from build123d import *

# Parameters (mm, degrees)
F1_W     = 50.8
F1_H     = 50.8
F3_W     = 50.8
F3_H     = 50.8
F4_DEPTH = 660.4


with BuildPart() as f2:
    # F2: sweep along a path in F0
    with BuildLine(Plane.XY) as f2_path:
        Line((0, 0), (0, 762))
        Line((0, 762), (1219.2, 762))
        Line((1219.2, 762), (1219.2, 0))
        Line((1219.2, 0), (0, 0))
    # F1 (on Front) → F2 (sweep)
    with BuildSketch(Plane.XZ):
        with Locations((25.4, -25.4)):
            Rectangle(F1_W, F1_H)
    sweep(path=f2_path.line, transition=Transition.RIGHT)

    # F3 (on face) → F4 (join, through all)
    with BuildSketch(Plane.XZ.offset(-711.2)):
        with Locations((990.6, -25.4)):
            Rectangle(F3_W, F3_H)
    extrude(amount=F4_DEPTH)


solid = f2.part
Source: CAD feature listing. Evaluate the final solid. Frame: model axes, mm. A direction names the side the tool comes from. Give positions to 0.01 mm unless a question says otherwise; leave off trailing zeros. Write each loop counter-clockwise with the first axis right and the second up, starting at its lowest first coordinate (ties: lowest second). Pieces come first, ordered by that corner, then holes. Notation, with made-up numbers: M 54.5,8.5 L 112.5,8.5 A16 cw 112.5,39.5 Z; hole C 68,-23.75 d1. An arc over 180 degrees is marked long. Return JSON: item names as keys, results as strings. Group by question number.
1) Set-up query: faces 5 (the face through (1093, 711.2, -26)), 6 (the face through (968, 383, -50.8)). Return all of +Z, -Z, +X, -X, +Y, -Y with unobstructed straight access to the full face (end or side cutting, diameter ignored); none if empty.
2) Cut plane B-B, the plane y = 316. Output: boundary loops of the cut face in (x, z).
3) Draft query along Y for faces 1 (the face through (974, 355, 0)), 2 (the face through (618, 762, -25)), 3 (the face through (601, 0, -25)), 4 (the face through (1016, 386, -26)). Return one class per face: released by +Y, released by -Y, zero draft, split by the parting line, or undercut.
4) Cut plane C-C, the plane z = -38. Output: boundary loops of the cut face in (x, y), then the cut area to 3 significant figures.
5) Ray query, L1, parallel to X at y = 213, z = -40.5; L2, parallel to Y at x = 572, z = -36.5. Return the intervals inside material, ascending.
6) Cut plane A-A, the plane x = 414. Output: boundary loops of the cut face in (y, z).
Data:
{
 "1": {"face 5": "+Z, -Z", "face 6": "-Z, +X, -X, +Y, -Y"},
 "2": {"outline": "M 0,-50.8 L 50.8,-50.8 L 50.8,0 L 0,0 Z; M 965.2,-50.8 L 1016,-50.8 L 1016,0 L 965.2,0 Z; M 1168.4,-50.8 L 1219.2,-50.8 L 1219.2,0 L 1168.4,0 Z"},
 "3": {"face 1": "zero draft", "face 2": "released by +Y", "face 3": "released by -Y", "face 4": "undercut"},
 "4": {"outline": "M 0,0 L 1219.2,0 L 1219.2,762 L 0,762 Z; hole M 50.8,50.8 L 965.2,50.8 L 965.2,711.2 L 50.8,711.2 Z; hole M 1016,50.8 L 1168.4,50.8 L 1168.4,711.2 L 1016,711.2 Z", "area": "225,000 mm²"},
 "5": {"L1": "x = 0 to 50.8, 965.2 to 1016, 1168.4 to 1219.2", "L2": "y = 0 to 50.8, 711.2 to 762"},
 "6": {"outline": "M 0,-50.8 L 50.8,-50.8 L 50.8,0 L 0,0 Z; M 711.2,-50.8 L 762,-50.8 L 762,0 L 711.2,0 Z"}
}
